Build history of the part. All positions in model axes, mm. Give positions to 0.01 mm unless a question says otherwise; leave off trailing zeros. Loops run counter-clockwise (first coordinate to the right, second up) from the corner with the lowest first, then second, coordinate; pieces in that order, holes last. Notation, with made-up numbers: (62, 17.25) -> (90, 17.25) arc R26 ccw to (90, 55.25) -> close; hole circle Ø11 at (86.25, 14.5). An arc over 180 degrees is marked (long way). Answer as a JSON object with one key per item and string values. Group by question number.
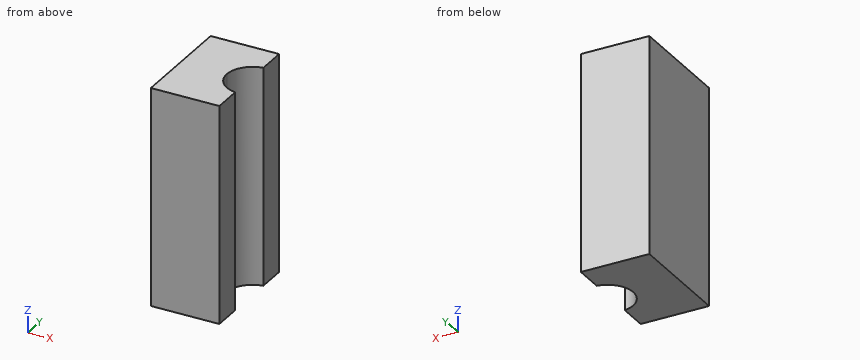
from build123d import *

# Parameters (mm, degrees)
F1_DEPTH = 25.4


with BuildPart() as f1:
    # F0 (on Top) → F1 (new body)
    with BuildSketch(Plane.XY):
        with BuildLine():
            Line((-2.625, 0), (-8, 0))
            Line((-8, 0), (-8, -6.35))
            Line((-8, -6.35), (0, -6.35))
            Line((0, -6.35), (0, -2.97647))
            ThreePointArc((0, -2.97647), (-1.875, -1.984313), (-2.625, 0))
        make_face()
        with BuildLine():
            Line((0, 6.35), (-8, 6.35))
            Line((-8, 6.35), (-8, 0))
            Line((-8, 0), (-2.625, 0))
            ThreePointArc((-2.625, 0), (-1.875, 1.984313), (0, 2.97647))
            Line((0, 2.97647), (0, 6.35))
        make_face()
    extrude(amount=F1_DEPTH)


solid = f1.part
(1) Saw through at B-B on z = 23. List the corners of the cut face in (x, y) (3 decimals).
(2) Probe line 1 along Y through (x, z) = (-0.25, 16.25); line 2 along Y through (x, z) = (-2, 10.25); line 3 along X through (y, z) = (-0.5, 21.25). List the from-to ranges inside material, lowest first. Write a range as [from, to].
(3) Saw through at C-C on y = -2.5. List the corners of the cut face in (x, z), plus the area to 3 significant figures.
(4) Pin check, flat tip, straight feed: pin 1 (1.5 mm diameter, centred on x = -3, y = 0.5, fed in from -Z). Stop position of the tip, or through.
(5) Saw through at A-A on x = -2. List the corners of the cut face in (y, z), plus the area to 3 significant figures.
(6) Saw through at D-D on y = -1. List the corners of the cut face in (x, z), plus the area to 3 significant figures.
Calculated:
{
 "1": {"outline": "(-8, -6.35) -> (0, -6.35) -> (0, -2.976) arc R3 cw to (-2.625, 0) arc R3 cw to (0, 2.976) -> (0, 6.35) -> (-8, 6.35) -> close"},
 "2": {"line 1": "y = [-6.35, -2.93], [2.93, 6.35]", "line 2": "y = [-6.35, -1.83], [1.83, 6.35]", "line 3": "x = [-8, -2.58]"},
 "3": {"outline": "(-8, 0) -> (-1.28, 0) -> (-1.28, 25.4) -> (-8, 25.4) -> close", "area": "171 mm^2"},
 "4": {"pin 1": "stops at z = 0"},
 "5": {"outline": "(-6.35, 0) -> (-1.83, 0) -> (-1.83, 25.4) -> (-6.35, 25.4) -> close; (1.83, 0) -> (6.35, 0) -> (6.35, 25.4) -> (1.83, 25.4) -> close", "area": "229 mm^2"},
 "6": {"outline": "(-8, 0) -> (-2.45, 0) -> (-2.45, 25.4) -> (-8, 25.4) -> close", "area": "141 mm^2"}
}
